```python
from build123d import *

# Parameters (mm, degrees)
BOSS_EXTRUDE1_DEPTH      = 6.35
BOSS_EXTRUDE3_DEPTH      = 11.43
BOSS_EXTRUDE3_DEPTH_BACK = 11.43
CUT_EXTRUDE13_DEPTH      = 55.124538916
CUT_EXTRUDE13_DEPTH_BACK = 55.124538916
SKETCH11_W               = 7.59470995
SKETCH11_H               = 29.201393096
CUT_EXTRUDE19_START      = -17.955569585
CUT_EXTRUDE19_DEPTH      = 17.955569585
SKETCH18_R               = 1.524
CUT_EXTRUDE22_DEPTH      = 58.631592142
CUT_EXTRUDE23_DEPTH      = 2.54
SKETCH22_R               = 1.524
CUT_EXTRUDE24_DEPTH      = 53.524026622
CUT_EXTRUDE25_DEPTH      = 2.54


# Read off the part's stored shape, not the designer's step: Cut-Extrude19
with BuildPart() as part:
    # Sketch1 → Boss-Extrude1 (new body)
    with BuildSketch(Plane(origin=(0, 0, 0), x_dir=(1, 0, 0), z_dir=(0, 1, 0))):
        with BuildLine():
            Line((11.43, 0), (11.43, -35.56))
            ThreePointArc((11.43, -35.56), (0, -46.99), (-11.43, -35.56))
            Line((-11.43, -35.56), (-11.43, 0))
            ThreePointArc((-11.43, 0), (0, 11.43), (11.43, 0))
        make_face()
    extrude(amount=-BOSS_EXTRUDE1_DEPTH)

    # Sketch2 → Boss-Extrude3 (add, two sides: drawn at the far end of the back side and taken through both)
    with BuildSketch(Plane(origin=(0, 0, 0), x_dir=(0, 0, -1), z_dir=(1, 0, 0)).offset(-BOSS_EXTRUDE3_DEPTH_BACK)):
        Polygon((-46.99, -6.35), (11.43, -6.35), (11.43, -9.525), (-11.11884122, -24.305569585), (-26.99384122, -24.305569585), (-46.99, -9.525), align=None)
    extrude(amount=BOSS_EXTRUDE3_DEPTH + BOSS_EXTRUDE3_DEPTH_BACK)

    # Sketch11 → Cut-Extrude13 (cut, two sides: drawn at the far end of the back side and taken through both)
    with BuildSketch(Plane.XY.offset(-CUT_EXTRUDE13_DEPTH_BACK)):
        with Locations((0.012645025, -20.950696548)):
            Rectangle(SKETCH11_W, SKETCH11_H)
    extrude(amount=CUT_EXTRUDE13_DEPTH + CUT_EXTRUDE13_DEPTH_BACK, mode=Mode.SUBTRACT)

    # Cut-Extrude19 outline → Cut-Extrude19 (cut)
    with BuildSketch(Plane(origin=(0, -6.35, 0), x_dir=(1, 0, 0), z_dir=(0, 1, 0)).offset(CUT_EXTRUDE19_START)):
        with BuildLine():
            Line((11.43, 11.43), (3.81, 11.43))
            Line((3.81, 11.43), (3.81, 10.776307345))
            ThreePointArc((3.81, 10.776307345), (9.33255592, 6.599113577), (11.43, 0))
            Line((11.43, 0), (11.43, 11.43))
        make_face()
        with BuildLine():
            ThreePointArc((11.43, -35.56), (9.332555866, -42.159113654), (3.809999822, -46.336307408))
            Line((3.809999822, -46.336307408), (3.81, -46.99))
            Line((3.81, -46.99), (11.43, -46.99))
            Line((11.43, -46.99), (11.43, -35.56))
        make_face()
        with BuildLine():
            ThreePointArc((-11.43, -5.66e-07), (-9.324809404, 6.610055188), (-3.78470995, 10.785215371))
            Line((-3.78470995, 10.785215371), (-3.78470995, 11.43))
            Line((-3.78470995, 11.43), (-11.43, 11.43))
            Line((-11.43, 11.43), (-11.43, -5.66e-07))
        make_face()
        with BuildLine():
            Line((-3.78470995, -46.99), (-3.784709773, -46.345215433))
            ThreePointArc((-3.784709773, -46.345215433), (-9.324809186, -42.170055495), (-11.43, -35.56))
            Line((-11.43, -35.56), (-11.43, -46.99))
            Line((-11.43, -46.99), (-3.78470995, -46.99))
        make_face()
    extrude(amount=CUT_EXTRUDE19_DEPTH, mode=Mode.SUBTRACT)

    # Sketch18 → Cut-Extrude22 (cut, through all)
    with BuildSketch(Plane.ZY.offset(11.43)):
        with Locations((19.062682441, -16.524127344)):
            Circle(SKETCH18_R)
    extrude(amount=-CUT_EXTRUDE22_DEPTH, mode=Mode.SUBTRACT)

    # Sketch20 → Cut-Extrude23 (cut)
    with BuildSketch(Plane.XZ.offset(6.35)):
        Polygon((0.016443108, 3.181298641), (-2.741372229, 1.60806008), (-2.757815336, -1.566897341), (-0.016443108, -3.1686162), (2.741372229, -1.595377639), (2.757815336, 1.579579782), align=None)
        Polygon((0.013747327, 34.440192786), (3.181851342, 36.285172538), (3.168104015, 39.951320972), (-0.013747327, 41.772489655), (-3.181851342, 39.927509903), (-3.168104015, 36.261361468), align=None)
    extrude(amount=-CUT_EXTRUDE23_DEPTH, mode=Mode.SUBTRACT)

    # Sketch22 → Cut-Extrude24 (cut, through all)
    with BuildSketch(Plane.XZ.offset(3.81)):
        with Locations(Location((0, 0, 0), (0, 0, 270))):
            Circle(SKETCH22_R)
        with Locations(Location((0, 38.094435686, 0), (0, 0, 270))):
            Circle(SKETCH22_R)
    extrude(amount=-CUT_EXTRUDE24_DEPTH, mode=Mode.SUBTRACT)

    # Sketch23 → Cut-Extrude25 (cut)
    with BuildSketch(Plane(origin=(11.43, 0, 0), x_dir=(0, 0, -1), z_dir=(1, 0, 0))):
        Polygon((-19.048935114, -20.190275778), (-15.880831099, -18.345296026), (-15.894578426, -14.679147592), (-19.076429768, -12.857978909), (-22.244533783, -14.702958661), (-22.230786456, -18.369107096), align=None)
    extrude(amount=-CUT_EXTRUDE25_DEPTH, mode=Mode.SUBTRACT)


solid = part.part
```
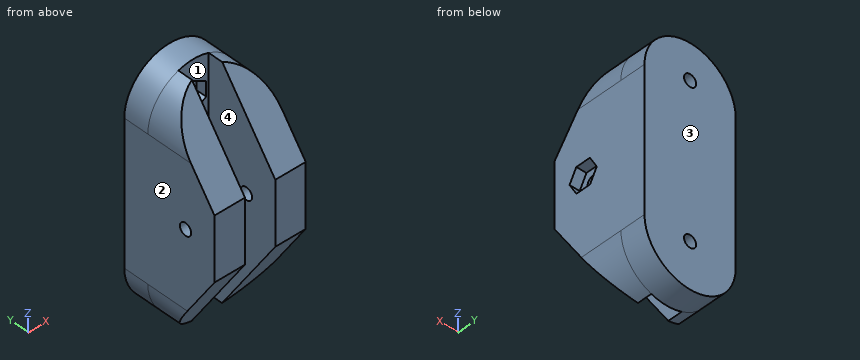
Part model, mm, in its own coordinate system. Face numbers are marked on the shaded views. Round coordinates to 2 decimals unless told otherwise and drop trailing zeros. Order: outer loops, then holes, each group sorted by start corner. A loop starts at its lowest first (then second) coordinate and runs counter-clockwise, first axis right, second up. Notation, with made-up numbers: M 48,27 L 65,27 A7 cw 65,34 Z; hole C 2,-4 d11. An arc over 180 degrees is marked long. Put each result on its own line as item: value. Start each with the question number.
1. Slice it at D-D on x = -7.5. List the corners of the cut face in (y, z), then the cut area to 3 significant figures.
2. Drill centre lines: probe 1 along X at (y, z) = (-12, 3); probe 2 along X at (y, z) = (-0.8, 0); probe 3 along Y at (x, z) = (-1, 12). Where is each one in solid material? Low to high. Write a range as [from, to].
3. Drop flat-ended pins along their axis: pin 1 (2.5 mm diameter, centred on y = -16.52, z = 19.06, fed in from -X); pin 2 (4 mm diameter, centred on x = -2, z = 32, fed in from -Y); pin 3 (5 mm diameter, centred on x = 4.5, z = 38.5, fed in from -Y); pin 4 (3 mm diameter, centred on x = 3, y = -15, fed in from -Z). Give the stop position or say it passes through.
4. Two-plate mould, pull along X, no slides. Class the marked faces 1, 2, 3 and 4: +X half, -X half, draft (parallel to the pull), parting line (faces both ways), or undercut.
5. Slice it at B-B on z = 14. List the corners of the cut face in (x, y), then the cut area to 3 significant figures.
6. Slice it at A-A on y = -2.25. List the corners of the cut face in (x, z), then the cut area to 3 significant figures.
7. Slice it at C-C on y = -11.5. List the corners of the cut face in (x, z).
Findings:
1. outline: M -24.31,11.12 L -11.36,-8.63 L 0,-8.63 L 0,44.19 L -11.6,44.19 L -24.31,26.99 Z; hole C -16.52,19.06 d3.05
1. area: 1,040 mm2
2. probe 1: [-11.43, -3.78], [3.81, 11.43]
2. probe 2: [-11.43, -1.52], [1.52, 11.43]
2. probe 3: [-6.35, 0]
3. pin 1: through
3. pin 2: y = -21.27
3. pin 3: y = -17.65
3. pin 4: z = -5
4. face 1: undercut
4. face 2: -X half
4. face 3: draft
4. face 4: undercut
5. outline: M -11.43,-24.31 L -3.78,-24.31 L -3.78,-6.35 L 3.81,-6.35 L 3.81,-24.31 L 11.43,-24.31 L 11.43,0 L -11.43,0 Z
5. area: 419 mm2
6. outline: M -11.43,0 A11.43 ccw 11.43,0 L 11.43,35.56 A11.43 ccw -11.43,35.56 Z; hole C 0,0 d3.05; hole C 0,38.09 d3.05
6. area: 1,210 mm2
7. outline: M -11.43,0 A11.43 ccw -7.73,-8.42 L -3.78,-8.42 L -3.78,44.32 L -7.34,44.32 A11.43 ccw -11.43,35.56 Z; M 3.81,-8.42 L 7.73,-8.42 A11.43 ccw 11.43,0 L 11.43,35.56 A11.43 ccw 7.34,44.32 L 3.81,44.32 Z
